```python
from build123d import *

# Parameters (mm, degrees)
SKETCH1_R           = 1.7272
SKETCH1_R_2         = 19.05
BOSS_EXTRUDE1_DEPTH = 6.35
BOSS_EXTRUDE2_START = 20.32
SKETCH3_R           = 29.251599278
SKETCH3_R_2         = 19.05
BOSS_EXTRUDE2_DEPTH = 20.32
FILLET1_R           = 3.175


with BuildPart() as part:
    # Sketch1 → Boss-Extrude1 (new body)
    with BuildSketch(Plane(origin=(0, 0, 0), x_dir=(0, 0, -1), z_dir=(1, 0, 0))):
        with BuildLine():
            ThreePointArc((30.954459577, 26.720579061), (16.530799639, 28.632184865), (7.663470482, 40.167637884))
            ThreePointArc((7.663470482, 40.167637884), (0, 46.0375), (-7.663470482, 40.167637884))
            ThreePointArc((-7.663470482, 40.167637884), (-16.530799639, 28.632184865), (-30.954459577, 26.720579061))
            ThreePointArc((-30.954459577, 26.720579061), (-39.869644527, 23.01875), (-38.617930059, 13.447058824))
            ThreePointArc((-38.617930059, 13.447058824), (-33.061599278, 0), (-38.617930059, -13.447058824))
            ThreePointArc((-38.617930059, -13.447058824), (-39.869644527, -23.01875), (-30.954459577, -26.720579061))
            ThreePointArc((-30.954459577, -26.720579061), (-16.530799639, -28.632184865), (-7.663470482, -40.167637884))
            ThreePointArc((-7.663470482, -40.167637884), (0, -46.0375), (7.663470482, -40.167637884))
            ThreePointArc((7.663470482, -40.167637884), (16.530799639, -28.632184865), (30.954459577, -26.720579061))
            ThreePointArc((30.954459577, -26.720579061), (39.869644527, -23.01875), (38.617930059, -13.447058824))
            ThreePointArc((38.617930059, -13.447058824), (33.061599278, 0), (38.617930059, 13.447058824))
            ThreePointArc((38.617930059, 13.447058824), (39.869644527, 23.01875), (30.954459577, 26.720579061))
        make_face()
        with Locations((-32.995567884, -19.05)):
            Circle(SKETCH1_R, mode=Mode.SUBTRACT)
        with Locations((0, -38.1)):
            Circle(SKETCH1_R, mode=Mode.SUBTRACT)
        with Locations((32.995567884, -19.05)):
            Circle(SKETCH1_R, mode=Mode.SUBTRACT)
        with Locations((-32.995567884, 19.05)):
            Circle(SKETCH1_R, mode=Mode.SUBTRACT)
        Circle(SKETCH1_R_2, mode=Mode.SUBTRACT)
        with Locations((32.995567884, 19.05)):
            Circle(SKETCH1_R, mode=Mode.SUBTRACT)
        with Locations((0, 38.1)):
            Circle(SKETCH1_R, mode=Mode.SUBTRACT)
    extrude(amount=BOSS_EXTRUDE1_DEPTH)

    # Sketch3 → Boss-Extrude2 (add)
    with BuildSketch(Plane.ZY.offset(BOSS_EXTRUDE2_START)):
        with Locations(Location((0, 0, 0), (0, 0, 180))):
            Circle(SKETCH3_R)
        with Locations(Location((0, 0, 0), (0, 0, 180))):
            Circle(SKETCH3_R_2, mode=Mode.SUBTRACT)
    extrude(amount=-BOSS_EXTRUDE2_DEPTH)

    # Fillet1
    fillet1_edges = [part.edges().sort_by_distance(p)[0] for p in [
        (0, 0, 29.251599278),
    ]]
    fillet(fillet1_edges, radius=FILLET1_R)

    # Mirror4: part across plane


with BuildPart() as part_1:
    add(part.part)
    add(part.part.mirror(Plane(origin=(-20.32, 0, 0), x_dir=(0, 0, 1), z_dir=(1, 0, 0))))


solid = part_1.part
```
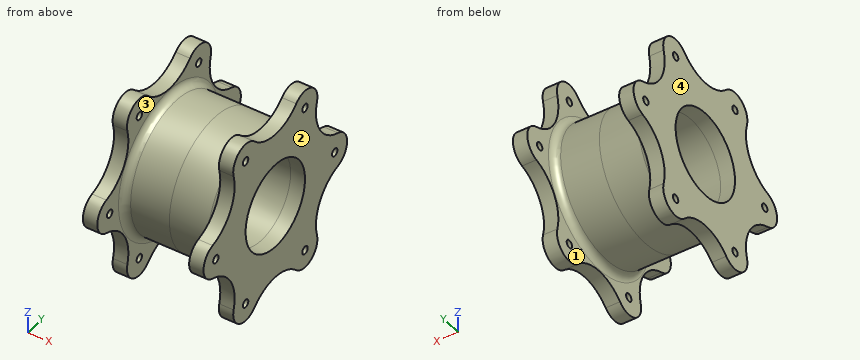
Read the model definition and answer for the solid it produces. Units are mm, in the model's axes. Face numbers are marked on the shaded views. Give positions to 0.01 mm unless a question says otherwise; leave off trailing zeros. Write each loop counter-clockwise with the first axis right and the second up, starting at its lowest first coordinate (ties: lowest second). Pieces come first, ordered by that corner, then holes. Notation, with made-up numbers: (-9, 62.5) -> (23, 62.5) arc R7 cw to (23, 69.5) -> close; hole circle Ø9 at (57, -38.5). An arc over 180 degrees is marked (long way). Answer in a Markdown table with one row per item.
1) Section C-C on z = 0 is taken. Count the separate pieces of the cut face and the enclosed holes in it, plus the area to 3 significant figures.
Results list:
| item | result |
|---|---|
| separate pieces | 6 |
| enclosed holes | 0 |
| area | 1,440 mm^2 |
2) Each of these flat-tipped pins is pushed along its axis until it touches: pin 1 Ø3 at (x, z) = (-21, 22.5) entering from +Y; pin 2 Ø6 at (x, z) = (-12, -9.5) entering from +Y; pin 3 Ø8 at (x, y) = (-9, 16.5) entering from -Z. Where does it stop, or does it pass through?
Results list:
| item | result |
|---|---|
| pin 1 | y = 20.36 |
| pin 2 | y = 28.52 |
| pin 3 | z = -26.45 |
3) Straight lines are drawn through the part: line 1 (X direction, y = -26, z = 24); line 2 (Y direction, x = -26, z = 0); line 3 (Z direction, x = -30, y = 9.5). For each, find the intervals that lie inside material, in ascending order. Write a range as [from, to].
Results list:
| item | result |
|---|---|
| line 1 | [-46.99, -40.64], [0, 6.35] |
| line 2 | [-29.25, -19.05], [19.05, 29.25] |
| line 3 | [-27.67, -16.51], [16.51, 27.67] |
4) Section A-A on y = 34 is taken. Give the vertices of the cut face in (x, z), plus the area to 3 significant figures.
Results list:
| item | result |
|---|---|
| outline | (-46.99, -10.6) -> (-40.64, -10.6) -> (-40.64, 10.6) -> (-46.99, 10.6) -> close; (0, -10.6) -> (6.35, -10.6) -> (6.35, 10.6) -> (0, 10.6) -> close |
| area | 269 mm^2 |
5) Section B-B on x = -8 is taken. Give the vertices of the cut face in (y, z).
Results list:
| item | result |
|---|---|
| outline | circle Ø58.5 at (0, 0); hole circle Ø38.1 at (0, 0) |
6) Determine the mould class of the marked faces 1, 2, 3 and 4 for opening direction X: released by +X, released by -X, zero draft, split by the parting line, or undercut.
Results list:
| item | result |
|---|---|
| face 1 | undercut |
| face 2 | released by +X |
| face 3 | undercut |
| face 4 | released by -X |
